Part model, mm, in its own coordinate system. A direction names the side the tool comes from. Round coordinates to 2 decimals unless told otherwise and drop trailing zeros. Loops run counter-clockwise (first coordinate to the right, second up) from the corner with the lowest first, then second, coordinate; pieces in that order, holes last. Notation, with made-up numbers: (-37, 70) - (-8, 70) arc R25 cw to (-8, 82) - close; hole circle Ø6 at (-7.75, 84.25). An arc over 180 degrees is marked (long way). Put each result on its own line as item: value.
from build123d import *

# Parameters (mm, degrees)
F2_DEPTH = 15
F3_R     = 36
F4_R     = 40
F5_R     = 2


with BuildPart() as f2:
    # F1 (on Right) → F2 (new body)
    with BuildSketch(Plane.YZ):
        with BuildLine():
            ThreePointArc((-7.6, -10.049876), (0, 12.6), (7.6, -10.049876))
            Line((7.6, -10.049876), (7.6, -33.003636))
            ThreePointArc((7.6, -33.003636), (27.035907, -47.332723), (34.976364, -24.528636))
            Line((34.976364, -24.528636), (30.850909, -27.353636))
            ThreePointArc((30.850909, -27.353636), (25.557272, -42.556361), (12.6, -33.003636))
            Line((12.6, -33.003636), (12.6, -12.288206))
            ThreePointArc((12.6, -12.288206), (0, 17.6), (-12.6, -12.288206))
            Line((-12.6, -12.288206), (-12.6, -33.003636))
            ThreePointArc((-12.6, -33.003636), (-25.557272, -42.556361), (-30.850909, -27.353636))
            Line((-30.850909, -27.353636), (-34.976364, -24.528636))
            ThreePointArc((-34.976364, -24.528636), (-27.035907, -47.332723), (-7.6, -33.003636))
            Line((-7.6, -33.003636), (-7.6, -10.049876))
        make_face()
    extrude(amount=F2_DEPTH)

    # F3
    f3_edges = [f2.edges().sort_by_distance(p)[0] for p in [
        (7.5, 12.6, -12.288206),
        (7.5, -12.6, -12.288206),
    ]]
    fillet(f3_edges, radius=F3_R)

    # F4
    f4_edges = [f2.edges().sort_by_distance(p)[0] for p in [
        (7.5, 7.6, -10.049876),
        (7.5, -7.6, -10.049876),
    ]]
    fillet(f4_edges, radius=F4_R)

    # F5
    f5_edges = [f2.edges().sort_by_distance(p)[0] for p in [
        (7.5, 30.850909, -27.353636),
        (7.5, 34.976364, -24.528636),
        (7.5, -30.850909, -27.353636),
        (7.5, -34.976364, -24.528636),
    ]]
    fillet(f5_edges, radius=F5_R)


solid = f2.part
1. Probe line 1 along Y through (x, z) = (3.25, -33); line 2 along Y through (x, z) = (11, -24); line 3 along Y through (x, z) = (4.75, 0). List the from-to ranges inside material, lowest first. Write a range as [from, to].
A:
line 1: y = [-37.6, -32.6], [-12.6, -7.6], [7.6, 12.6], [32.6, 37.6]
line 2: y = [-12.6, -7.6], [7.6, 12.6]
line 3: y = [-17.6, -12.6], [12.6, 17.6]
2. Band-saw the part on A-A (z = -12). List the corners of the cut face in (x, y).
A:
outline: (0, -14.2) - (15, -14.2) - (15, -8.97) - (0, -8.97) - close; (0, 8.97) - (15, 8.97) - (15, 14.2) - (0, 14.2) - close
3. Pin check, flat tips, straight feed: P1, Ø5.5, axis at x = 8, z = -28, coming from the +Y side; P2, Ø8, axis at x = 11.5, z = -14.5, coming from the -Y side; P3, Ø12, axis at y = 22.6, z = -33, coming from the +X side; P4, Ø5, axis at x = 9.5, z = -17, coming from the -Y side. Stop position of each tip, or through.
A:
P1: stops at y = 37.43
P2: stops at y = -14.7
P3: passes through
P4: stops at y = -13.52
4. Band-saw the part on D-D (x = 11.25). List the corners of the cut face in (y, z).
A:
outline: (-36.13, -26.53) arc R15 ccw (long way) to (-7.6, -33) - (-7.6, -22.38) arc R40 ccw to (-11.4, -5.36) arc R12.6 cw (long way) to (11.4, -5.36) arc R40 ccw to (7.6, -22.38) - (7.6, -33) arc R15 ccw (long way) to (36.13, -26.53) arc R2 ccw to (33.2, -25.75) - (32.36, -26.32) arc R2 ccw to (31.68, -28.81) arc R10 cw (long way) to (12.6, -33) - (12.6, -22.61) arc R36 cw to (15.96, -7.42) arc R17.6 ccw (long way) to (-15.96, -7.42) arc R36 cw to (-12.6, -22.61) - (-12.6, -33) arc R10 cw (long way) to (-31.68, -28.81) arc R2 ccw to (-32.36, -26.32) - (-33.2, -25.75) arc R2 ccw to start
5. Band-saw the part on C-C (y = 22.6). List the corners of the cut face in (x, z), plus the area to 3 significant figures.
A:
outline: (0, -48) - (15, -48) - (15, -43) - (0, -43) - close
area: 75.0 mm²
6. Two-plate mould, pull along Z, no slides. Class faces 5 (the cylindrical face through (7.4, -24.5, -42.82)), 6 (the flat face through (0, 8, -22)), 7 (the cylindrical face through (7.6, 34.87, -25.47)): pulls with the +Z half, pulls with the -Z half, needs draft (parallel to the pull), parting line crosses it, or undercut.
A:
face 5: undercut
face 6: needs draft
face 7: pulls with the +Z half
7. Tool access for faces 1 (the cylindrical face through (7.605, -13.473, -14.723)), 2 (the cylindrical face through (7.605, 13.426, -14.938)), 3 (the cylindrical face through (7.6, -8.6, -13.5)), 4 (the flat face through (7, -7.6, -28)): list every direction of +Z, -Z, +X, -X, +Y, -Y with a clear straight run to the whole face (end or side of a thin tool).
A:
face 1: +X, -X, -Y
face 2: +X, -X, +Y
face 3: +X, -X
face 4: -Z, +X, -X
8. Band-saw the part on B-B (z = -35). List the corners of the cut face in (x, y).
A:
outline: (0, -37.47) - (15, -37.47) - (15, -32.4) - (0, -32.4) - close; (0, -12.8) - (15, -12.8) - (15, -7.73) - (0, -7.73) - close; (0, 7.73) - (15, 7.73) - (15, 12.8) - (0, 12.8) - close; (0, 32.4) - (15, 32.4) - (15, 37.47) - (0, 37.47) - close
